Answer from the drawing. Dimensions are ordinates in mm from the lowest x, y and z of the part. A direction names the side the tool comes from. Coordinates: 2 decimals unless noted, no trailing zeros. Order: outer loops, then holes, each group sorted by start corner. A loop starts at its lowest first (then second) coordinate and runs counter-clockwise, first axis right, second up.
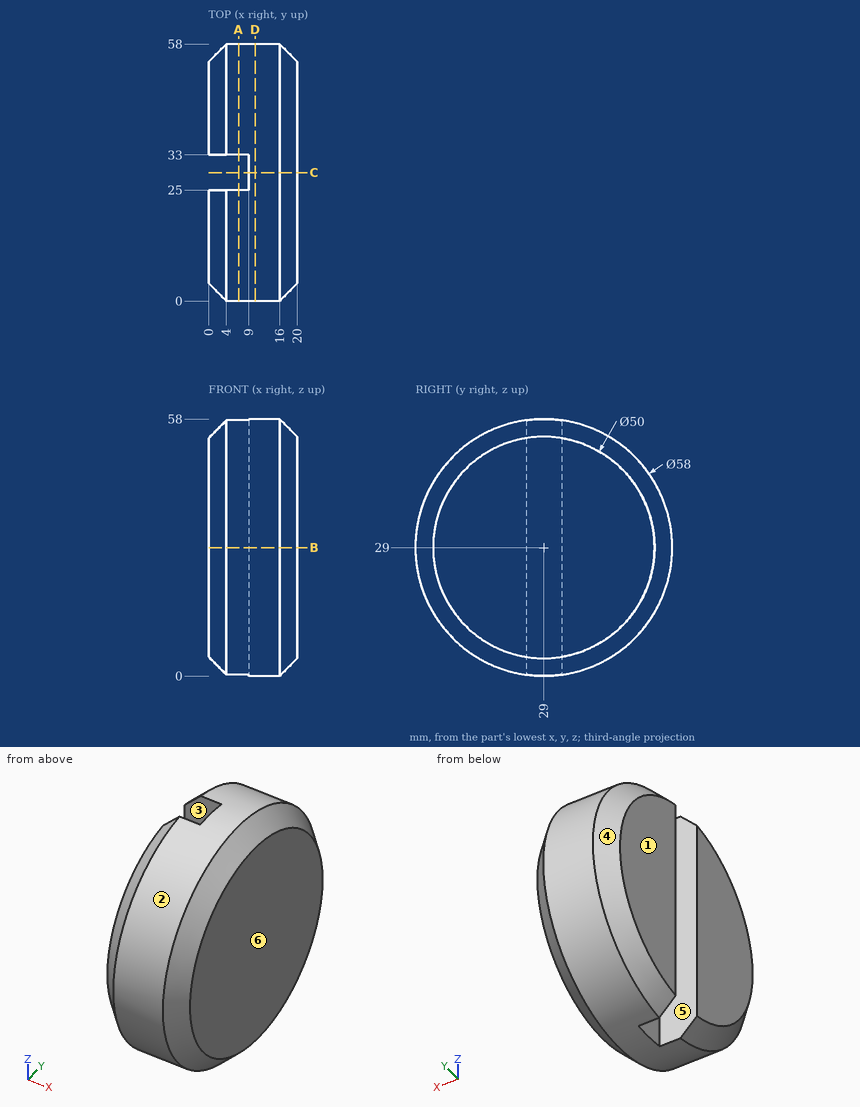
1. The part is cut by section D-D (x = 10.5). Determine the outline of the cut face in (y, z).
2. For the marked faces 5 and 6, determine the directions among +Z, -Z, +X, -X, +Y, -Y from which every point of the face is accessible in a straight line to the end or side of a thin tool.
3. The part is cut by section A-A (x = 6.75). Determine the outline of the cut face in (y, z).
4. The part is cut by section B-B (z = 29). Determine the outline of the cut face in (x, y), plus the area to 3 significant figures.
5. Flat-ended cylindrical pins translate along their axes: pin 1 (6.5 mm diameter, centred on y = 28.5, z = 21.5, fed in from -X); pin 2 (2 mm diameter, centred on x = 11.5, y = 11.5, fed in from +Z); pin 3 (12 mm diameter, centred on x = 9.5, z = 32.5, fed in from -Y); pin 4 (4 mm diameter, centred on x = 12, y = 7, fed in from -Z). Find the tip coordinate at first contact, or state that the pin passes through.
6. The part is cut by section C-C (y = 29). Determine the outline of the cut face in (x, z).
7. The mould has two halves that part along Y. Classify the marked faces 1, 2, 3 and 4: released by +Y, released by -Y, zero draft, split by the parting line, or undercut.
8. Consider probe 1 along Y at (x, z) = (12.25, 25); probe 2 along Y at (x, z) = (8.25, 44); probe 3 along Y at (x, z) = (1.25, 32). Determine where each line is inside the solid, lowest interval first.
Worked out:
1. outline: circle Ø58 at (29, 29)
2. face 5: +Z, -Z, -X
2. face 6: +Z, -Z, +X, +Y, -Y
3. outline: (25, 0.28) - (25, 57.72) arc R29 ccw to start; (33, 0.28) arc R29 ccw to (33, 57.72) - close
4. outline: (0, 4) - (4, 0) - (16, 0) - (20, 4) - (20, 54) - (16, 58) - (4, 58) - (0, 54) - (0, 33) - (9, 33) - (9, 25) - (0, 25) - close
4. area: 1,060 mm2
5. pin 1: stops at x = 9
5. pin 2: stops at z = 52.85
5. pin 3: stops at y = 0
5. pin 4: stops at z = 8
6. outline: (9, 0) - (16, 0) - (20, 4) - (20, 54) - (16, 58) - (9, 58) - close
7. face 1: zero draft
7. face 2: split by the parting line
7. face 3: undercut
7. face 4: released by +Y
8. probe 1: y = 0.28 to 57.72
8. probe 2: y = 4.18 to 25, 33 to 53.82
8. probe 3: y = 2.92 to 25, 33 to 55.08
